from build123d import *

# Parameters (mm, degrees)
CUT_EXTRUDE_8_DEPTH      = 184.806963974
EXTRUDE_1_DEPTH          = 9
EXTRUDE_1_DEPTH_BACK     = 9
EXTRUDE_2_DEPTH          = 3
EXTRUDE_2_DEPTH_BACK     = 3
SKETCH_2_R               = 13
SKETCH_2_R_2             = 13.100880905
CUT_EXTRUDE_7_DEPTH      = 190.570567491
CUT_EXTRUDE_9_DEPTH      = 190.570567491
CUT_EXTRUDE_9_DEPTH_BACK = 190.570567491
CHAMFER_4_SIZE           = 2
CHAMFER_5_SIZE           = 2
CHAMFER_6_SIZE           = 2


with BuildPart() as part:
    # Sketch 1 → Revolve 1 (revolve)
    with BuildSketch(Plane.XY, mode=Mode.PRIVATE) as revolve_1_sk:
        with BuildLine():
            Line((-62, 2), (-62, 138))
            ThreePointArc((-62, 138), (-62.585786438, 139.414213562), (-64, 140))
            Line((-64, 140), (-89, 140))
            Line((-89, 140), (-89, 0))
            Line((-89, 0), (-64, 0))
            ThreePointArc((-64, 0), (-62.585786438, 0.585786438), (-62, 2))
        make_face()
    revolve(revolve_1_sk.sketch.rotate(Axis((-89, 140, 0), (0, -1, 0)), 180), axis=Axis((-89, 140, 0), (0, -1, 0)))

    # Sketch 5 → Cut-Extrude 8 (cut, through all)
    with BuildSketch(Plane.XY):
        with BuildLine():
            Line((-116, 115), (-41, 115))
            ThreePointArc((-41, 115), (-39.585786438, 114.414213562), (-39, 113))
            Line((-39, 113), (-39, 52))
            ThreePointArc((-39, 52), (-39.585786438, 50.585786438), (-41, 50))
            Line((-41, 50), (-116, 50))
            Line((-116, 50), (-116, 115))
        make_face()
        with BuildLine():
            Line((50, 79.693161564), (50, 60))
            ThreePointArc((50, 60), (49.414213562, 58.585786438), (48, 58))
            Line((48, 58), (-23, 58))
            ThreePointArc((-23, 58), (-24.414213562, 58.585786438), (-25, 60))
            Line((-25, 60), (-25, 121.655250606))
            ThreePointArc((-25, 121.655250606), (-24.27000127, 123.200273834), (-22.612903226, 123.617432067))
            ThreePointArc((-22.612903226, 123.617432067), (17.108435299, 108.471694573), (49.532258065, 80.978535137))
            ThreePointArc((49.532258065, 80.978535137), (49.87943025, 80.377078178), (50, 79.693161564))
        make_face()
    extrude(amount=-CUT_EXTRUDE_8_DEPTH, mode=Mode.SUBTRACT)



with BuildPart() as body_2:
    # Sketch 1_4 → Revolve 2 (revolve)
    with BuildSketch(Plane.XY, mode=Mode.PRIVATE) as revolve_2_sk:
        with BuildLine():
            Line((62, 2), (62, 106))
            ThreePointArc((62, 106), (64.050252532, 110.949747468), (69, 113))
            Line((69, 113), (93, 113))
            Line((93, 113), (93, 0))
            Line((93, 0), (64, 0))
            ThreePointArc((64, 0), (62.585786438, 0.585786438), (62, 2))
        make_face()
    revolve(revolve_2_sk.sketch.rotate(Axis((93, 113, 0), (0, -1, 0)), 270), axis=Axis((93, 113, 0), (0, -1, 0)))


with BuildPart() as part_1:
    add(part.part)

    add(body_2.part)  # Extrude 1 merges body 2
    # Sketch 1_5 → Extrude 1 (add, two sides: drawn at the far end of the back side and taken through both)
    # profile 1 of 3: a face of its own
    with BuildSketch(Plane.XY.offset(-EXTRUDE_1_DEPTH_BACK)):
        with BuildLine():
            ThreePointArc((-62, 2), (-62.585786438, 0.585786438), (-64, 0))
            Line((-64, 0), (-47, 0))
            Line((-47, 0), (64, 0))
            ThreePointArc((64, 0), (62.585786438, 0.585786438), (62, 2))
            Line((62, 2), (62, 87.857839718))
            ThreePointArc((62, 87.857839718), (13.414826158, 126.293502526), (-47, 140))
            Line((-47, 140), (-64, 140))
            ThreePointArc((-64, 140), (-62.585786438, 139.414213562), (-62, 138))
            Line((-62, 138), (-62, 2))
        make_face()
        with BuildLine():
            Line((56, 6), (-47, 6))
            Line((-47, 6), (-55, 6))
            ThreePointArc((-55, 6), (-56.414213562, 6.585786438), (-57, 8))
            Line((-57, 8), (-57, 132))
            ThreePointArc((-57, 132), (-56.414213562, 133.414213562), (-55, 134))
            Line((-55, 134), (-47, 134))
            ThreePointArc((-47, 134), (10.992622758, 120.800892818), (57.560606061, 83.803816502))
            ThreePointArc((57.560606061, 83.803816502), (57.886956825, 83.215881236), (58, 82.55301327))
            Line((58, 82.55301327), (58, 8))
            ThreePointArc((58, 8), (57.414213562, 6.585786438), (56, 6))
        make_face(mode=Mode.SUBTRACT)
    # profile 2 of 3: a face of its own
    with BuildSketch(Plane.XY.offset(-EXTRUDE_1_DEPTH_BACK)):
        with BuildLine():
            Line((-89, 0), (-64, 0))
            ThreePointArc((-64, 0), (-62.585786438, 0.585786438), (-62, 2))
            Line((-62, 2), (-62, 138))
            ThreePointArc((-62, 138), (-62.585786438, 139.414213562), (-64, 140))
            Line((-64, 140), (-89, 140))
            Line((-89, 140), (-89, 0))
        make_face()
    # profile 3 of 3: a face of its own
    with BuildSketch(Plane.XY.offset(-EXTRUDE_1_DEPTH_BACK)):
        with BuildLine():
            ThreePointArc((62, 2), (62.585786438, 0.585786438), (64, 0))
            Line((64, 0), (93, 0))
            ThreePointArc((93, 0), (85.022725317, 46.583258795), (62, 87.857839718))
            Line((62, 87.857839718), (62, 2))
        make_face()
    extrude(amount=EXTRUDE_1_DEPTH + EXTRUDE_1_DEPTH_BACK)

    # Sketch 1_6 → Extrude 2 (add, two sides: drawn at the far end of the back side and taken through both)
    with BuildSketch(Plane.XY.offset(-EXTRUDE_2_DEPTH_BACK)):
        with BuildLine():
            Line((-47, 134), (-47, 6))
            Line((-47, 6), (56, 6))
            ThreePointArc((56, 6), (57.414213562, 6.585786438), (58, 8))
            Line((58, 8), (58, 82.55301327))
            ThreePointArc((58, 82.55301327), (57.886956825, 83.215881236), (57.560606061, 83.803816502))
            ThreePointArc((57.560606061, 83.803816502), (10.992622758, 120.800892818), (-47, 134))
        make_face()
        with BuildLine():
            Line((-55, 6), (-47, 6))
            Line((-47, 6), (-47, 134))
            Line((-47, 134), (-55, 134))
            ThreePointArc((-55, 134), (-56.414213562, 133.414213562), (-57, 132))
            Line((-57, 132), (-57, 8))
            ThreePointArc((-57, 8), (-56.414213562, 6.585786438), (-55, 6))
        make_face()
    extrude(amount=EXTRUDE_2_DEPTH + EXTRUDE_2_DEPTH_BACK)

    # Sketch 2 → Cut-Extrude 7 (cut, through all)
    with BuildSketch(Plane(origin=(0, 0, 0), x_dir=(1, 0, 0), z_dir=(0, 1, 0))):
        with Locations(Location((-89, 0, 0), (0, 0, 270))):
            Circle(SKETCH_2_R)
        with Locations(Location((93, 0, 0), (0, 0, 90))):
            Circle(SKETCH_2_R_2)
    extrude(amount=CUT_EXTRUDE_7_DEPTH, mode=Mode.SUBTRACT)

    # Sketch 5_2 → Cut-Extrude 9 (cut, two sides: drawn at the far end of the back side and taken through both)
    with BuildSketch(Plane.XY.offset(-CUT_EXTRUDE_9_DEPTH_BACK)):
        with BuildLine():
            Line((-116, 115), (-41, 115))
            ThreePointArc((-41, 115), (-39.585786438, 114.414213562), (-39, 113))
            Line((-39, 113), (-39, 52))
            ThreePointArc((-39, 52), (-39.585786438, 50.585786438), (-41, 50))
            Line((-41, 50), (-116, 50))
            Line((-116, 50), (-116, 115))
        make_face()
        with BuildLine():
            Line((50, 79.693161564), (50, 60))
            ThreePointArc((50, 60), (49.414213562, 58.585786438), (48, 58))
            Line((48, 58), (-23, 58))
            ThreePointArc((-23, 58), (-24.414213562, 58.585786438), (-25, 60))
            Line((-25, 60), (-25, 121.655250606))
            ThreePointArc((-25, 121.655250606), (-24.27000127, 123.200273834), (-22.612903226, 123.617432067))
            ThreePointArc((-22.612903226, 123.617432067), (17.108435299, 108.471694573), (49.532258065, 80.978535137))
            ThreePointArc((49.532258065, 80.978535137), (49.87943025, 80.377078178), (50, 79.693161564))
        make_face()
    extrude(amount=CUT_EXTRUDE_9_DEPTH + CUT_EXTRUDE_9_DEPTH_BACK, mode=Mode.SUBTRACT)

    # Chamfer 4
    chamfer_4_edges = [part_1.edges().sort_by_distance(p)[0] for p in [
        (93, 0, 13.100880905),
        (93, 113, 13.100880905),
    ]]
    chamfer(chamfer_4_edges, length=CHAMFER_4_SIZE)

    # Chamfer 5
    chamfer_5_edges = [part_1.edges().sort_by_distance(p)[0] for p in [
        (-89, 115, -13),
        (-89, 140, -13),
    ]]
    chamfer(chamfer_5_edges, length=CHAMFER_5_SIZE)

    # Chamfer 6
    chamfer_6_edges = [part_1.edges().sort_by_distance(p)[0] for p in [
        (-89, 0, -13),
        (-89, 50, -13),
    ]]
    chamfer(chamfer_6_edges, length=CHAMFER_6_SIZE)


solid = part_1.part
Can you work these out from the model? Positions are in its coordinate system, mm. A direction names the side the tool comes from. Give positions to 0.01 mm unless a question says otherwise; leave off trailing zeros. Order: outer loops, then holes, each group sorted by start corner. A loop starts at its lowest first (then second) coordinate and runs counter-clockwise, first axis right, second up. Notation, with made-up numbers: M -34,10 L -3,10 A30 cw -3,37 Z; hole C 56.25,52.25 d7. An arc over 180 degrees is marked long. One line per item, written item: value.
Item 1: For pin 1 (3 mm diameter, centred on x = 11, y = 122, fed in from +Z); pin 2 (3 mm diameter, centred on y = 41, z = 7.5, fed in from -X); pin 3 (6.5 mm diameter, centred on y = 31.5, z = -5.5, fed in from +X), each with a flat end and sliding along its axis, tell me the tip position at first contact or that it passes through.
Verdict:
pin 1: z = 9
pin 2: x = -115.32
pin 3: x = 123.92
Item 2: Please list where these lines run through material, in increasing order: line 1 (X direction, y = 39, z = 0); line 2 (X direction, y = 60.5, z = 0); line 3 (Z direction, x = 93, y = 59).
Verdict:
line 1: -116 to -102, -76 to 79.9, 106.1 to 124
line 2: -39 to -25, 50 to 79.9, 106.1 to 124
line 3: -31 to -13.1, 13.1 to 31
Item 3: If we mould it in two halves opening along Y, with no side actions, what happens to faces 1 (the face through (43, 101, 9)), 2 (the face through (-57, 29, 6)), 3 (the face through (109, 113, 0))? For each: pulls with the +Y half, pulls with the -Y half, needs draft (parallel to the pull), parting line crosses it, or undercut.
Verdict:
face 1: needs draft
face 2: undercut
face 3: pulls with the +Y half
Item 4: If we section it at D-D on y = 15: Write out the boundary of the cut face in (x, z).
Verdict:
outline: M -63.54,-9 L -57,-9 L -57,-3 L 58,-3 L 58,-9 L 63.34,-9 A31 ccw long 63.34,9 L 58,9 L 58,3 L -57,3 L -57,9 L -63.54,9 A27 ccw long Z; hole C -89,0 d26; hole C 93,0 d26.2
Item 5: If we section it at C-C on x = 93: Write out the boundary of the cut face in (y, z).
Verdict:
outline: M 0,-29 A2 ccw 2,-31 L 106,-31 A7 ccw 113,-24 L 113,-15.1 L 111,-13.1 L 2,-13.1 L 0,-15.1 Z; M 0,15.1 L 2,13.1 L 111,13.1 L 113,15.1 L 113,24 A7 ccw 106,31 L 2,31 A2 ccw 0,29 Z
Item 6: For faces 4 (the face through (-51, 134, 6)), 5 (the face through (10.235, 121.162, -6.042)), 6 (the face through (50, 70, 0)), 7 (the face through (-78, 50, -12)), which set-ups out of +Z, -Z, +X, -X, +Y, -Y let a thin tool reach every point of the face, with its end or its side?
Verdict:
face 4: +Z
face 5: -Z
face 6: +Z, -Z
face 7: +Z, -Z, -X
Item 7: If we section it at B-B on y = 63.5: Write out the boundary of the cut face in (x, z).
Verdict:
outline: M -39,-3 L -25,-3 L -25,3 L -39,3 Z; M 50,-3 L 58,-3 L 58,-9 L 63.34,-9 A31 ccw long 63.34,9 L 58,9 L 58,3 L 50,3 Z; hole C 93,0 d26.2
Item 8: If we section it at A-A on x = -89: Write out the boundary of the cut face in (y, z).
Verdict:
outline: M 0,-25 A2 ccw 2,-27 L 50,-27 L 50,-15 L 48,-13 L 2,-13 L 0,-15 Z; M 0,15 L 2,13 L 48,13 L 50,15 L 50,27 L 2,27 A2 ccw 0,25 Z; M 115,-27 L 138,-27 A2 ccw 140,-25 L 140,-15 L 138,-13 L 117,-13 L 115,-15 Z; M 115,15 L 117,13 L 138,13 L 140,15 L 140,25 A2 ccw 138,27 L 115,27 Z
